from build123d import *

# Parameters (mm, degrees)
SKETCH1_W           = 139.73
SKETCH1_H           = 31.67
BOSS_EXTRUDE1_DEPTH = 19.5
SKETCH2_W           = 139.73
SKETCH2_H           = 25.71
CUT_EXTRUDE1_DEPTH  = 17.97
HOLE1_D             = 4.84
HOLE1_DEPTH         = 2.98
HOLE2_D             = 6.06
HOLE2_DEPTH         = 1.53


with BuildPart() as part:
    # Sketch1 → Boss-Extrude1 (new body)
    with BuildSketch(Plane(origin=(0, 0, 0), x_dir=(1, 0, 0), z_dir=(0, 1, 0))):
        with Locations((69.865, -15.835)):
            Rectangle(SKETCH1_W, SKETCH1_H)
    extrude(amount=BOSS_EXTRUDE1_DEPTH)

    # Sketch2 → Cut-Extrude1 (cut)
    with BuildSketch(Plane.XZ):
        with Locations((69.865, 15.835)):
            Rectangle(SKETCH2_W, SKETCH2_H)
    extrude(amount=-CUT_EXTRUDE1_DEPTH, mode=Mode.SUBTRACT)

    # Hole1
    with Locations(Plane(origin=(0, 0, 0), x_dir=(-1, 0, 0), z_dir=(0, 0, -1))):
        with Locations((-131.3, 3.93), (-96.59, 3.93), (-43.14, 3.93), (-8.43, 3.93)):
            Hole(HOLE1_D / 2, depth=HOLE1_DEPTH)

    # Hole2
    with Locations(Plane(origin=(0, 19.5, 0), x_dir=(-1, 0, 0), z_dir=(0, 1, 0))):
        with Locations((-122.87, 21.38), (-106.26, 21.38), (-33.38, 21.38), (-17.32, 21.38)):
            Hole(HOLE2_D / 2, depth=HOLE2_DEPTH)


solid = part.part
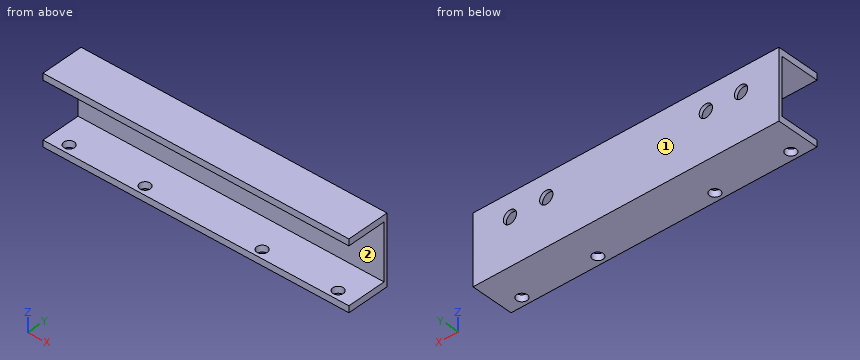
For this review, take the finished solid that the model builds, in its own axes (mm). Face numbers are marked on the shaded views. A direction names the side the tool comes from. Round coordinates to 2 decimals unless told otherwise and drop trailing zeros. Write each loop counter-clockwise with the first axis right and the second up, starting at its lowest first coordinate (ties: lowest second). Pieces come first, ordered by that corner, then holes. Notation, with made-up numbers: (29, 61) -> (77, 61) arc R35 cw to (77, 97) -> close; hole circle Ø6 at (72.25, 73.25). An arc over 180 degrees is marked (long way). Put each result on its own line as item: value.
Q1. Consider section B-B on z = 21.38. State the section outline as (x, y) points, and give its area (3 significant figures).
Determined:
outline: (0, 17.97) -> (14.29, 17.97) -> (14.29, 19.5) -> (0, 19.5) -> close; (20.35, 17.97) -> (30.35, 17.97) -> (30.35, 19.5) -> (20.35, 19.5) -> close; (36.41, 17.97) -> (103.23, 17.97) -> (103.23, 19.5) -> (36.41, 19.5) -> close; (109.29, 17.97) -> (119.84, 17.97) -> (119.84, 19.5) -> (109.29, 19.5) -> close; (125.9, 17.97) -> (139.73, 17.97) -> (139.73, 19.5) -> (125.9, 19.5) -> close
area: 177 mm^2
Q2. Machinability: for the marked faces 1 and 2, which of the approach directions +Z, -Z, +X, -X, +Y, -Y give a long, thin tool a straight path to every point of the face, cutting with its end or side? Answer none if there is none.
Determined:
face 1: +Z, -Z, +X, -X, +Y
face 2: +X, -X, -Y
Q3. Consider section A-A on x = 131.3. State the section outline as (y, z) points, and give its area (3 significant figures).
Determined:
outline: (0, 0) -> (1.51, 0) -> (1.51, 2.98) -> (0, 2.98) -> close; (0, 28.69) -> (17.97, 28.69) -> (17.97, 2.98) -> (6.35, 2.98) -> (6.35, 0) -> (19.5, 0) -> (19.5, 31.67) -> (0, 31.67) -> close
area: 141 mm^2
Q4. Clearance check with flat-ended pins moving along their axes: pin 1 Ø7 at (x, z) = (106.26, 21.38) entering from -Y; pin 2 Ø4.5 at (x, y) = (43.14, 3.93) entering from -Z. State where each tip first meets the part, or that it passes through.
Determined:
pin 1: stops at y = 17.97
pin 2: stops at z = 28.69
Q5. To check wall thickness, follow L1, parallel to Z at x = 33.38, y = 18.45; L2, parallel to Z at x = 60.5, y = 11.25; L3, parallel to X at y = 6, z = 2. State the ranges of each line that lie inside material, in increasing order. Write a range as [from, to].
Determined:
L1: z = [0, 18.35], [24.41, 31.67]
L2: z = [0, 2.98], [28.69, 31.67]
L3: x = [0, 7.18], [9.68, 41.89], [44.39, 95.34], [97.84, 130.05], [132.55, 139.73]
Q6. Consider section C-C on x = 57. State the section outline as (y, z) points.
Determined:
outline: (0, 0) -> (19.5, 0) -> (19.5, 31.67) -> (0, 31.67) -> (0, 28.69) -> (17.97, 28.69) -> (17.97, 2.98) -> (0, 2.98) -> close
Q7. Consider section D-D on z = 7.5. State the section outline as (x, y) points.
Determined:
outline: (0, 17.97) -> (139.73, 17.97) -> (139.73, 19.5) -> (0, 19.5) -> close
